```python
from build123d import *

# Parameters (mm, degrees)
SKETCH_W     = 120
SKETCH_H     = 80
PAD_DEPTH    = 20
SKETCH001_R  = 20
POCKET_DEPTH = 20


with BuildPart() as part:
    # Sketch → Pad (new body)
    with BuildSketch(Plane.XY):
        Rectangle(SKETCH_W, SKETCH_H)
    extrude(amount=PAD_DEPTH)

    # Sketch001 (on Face6 of Pad) → Pocket (cut)
    with BuildSketch(Plane.XY.offset(20)):
        Circle(SKETCH001_R)
    extrude(amount=-POCKET_DEPTH, mode=Mode.SUBTRACT)


solid = part.part
```
Model file for the job. Use its own axes, mm. Round coordinates to 2 decimals unless told otherwise and drop trailing zeros. Write each loop counter-clockwise with the first axis right and the second up, starting at its lowest first coordinate (ties: lowest second). Pieces come first, ordered by that corner, then holes. Notation, with made-up numbers: (-2, 85.5) -> (47, 85.5) arc R25 cw to (47, 108.5) -> close; hole circle Ø5 at (27, 88.5). An arc over 180 degrees is marked (long way). Answer as CSV lines item,"result".
1. Slice it at C-C, the plane z = 2. List the corners of the cut face in (x, y), plus the area to 3 significant figures.
Resolved:
outline,"(-60, -40) -> (60, -40) -> (60, 40) -> (-60, 40) -> close; hole circle Ø40 at (0, 0)"
area,"8,340 mm²"
2. Slice it at B-B, the plane y = 0. List the corners of the cut face in (x, z), plus the area to 3 significant figures.
Resolved:
outline,"(-60, 0) -> (-20, 0) -> (-20, 20) -> (-60, 20) -> close; (20, 0) -> (60, 0) -> (60, 20) -> (20, 20) -> close"
area,"1,600 mm²"
3. Drill centre lines: line 1 (Y direction, x = 0, z = 7); line 2 (X direction, y = -6, z = 7.5); line 3 (Y direction, x = -7, z = 10) (3 decimals). Where is each one in solid material? Low to high.
Resolved:
line 1,"-40 to -20, 20 to 40"
line 2,"-60 to -19.08, 19.08 to 60"
line 3,"-40 to -18.735, 18.735 to 40"
4. Mould opens along Y. For faces 1 (the face through (-14, 18, 20)), 2 (the face through (-1, 40, 10)), 3 (the face through (-4.336, -19.524, 10.14)), 4 (the face through (-1, -40, 10)) say: +Y half, -Y half, draft (parallel to the pull), parting line (faces both ways), or undercut.
Resolved:
face 1,"draft"
face 2,"+Y half"
face 3,"undercut"
face 4,"-Y half"
5. Slice it at A-A, the plane x = 0. List the corners of the cut face in (y, z), plus the area to 3 significant figures.
Resolved:
outline,"(-40, 0) -> (-20, 0) -> (-20, 20) -> (-40, 20) -> close; (20, 0) -> (40, 0) -> (40, 20) -> (20, 20) -> close"
area,"800 mm²"
6. Pin check, flat tip, straight feed: pin 1 Ø8 at (x, y) = (25, -28.5) entering from -Z. Stop position of the tip, or through.
Resolved:
pin 1,"z = 0"
